Part model, mm, in its own coordinate system. Face numbers are marked on the shaded views. A direction names the side the tool comes from. Round coordinates to 2 decimals unless told otherwise and drop trailing zeros. Loops run counter-clockwise (first coordinate to the right, second up) from the corner with the lowest first, then second, coordinate; pieces in that order, holes last. Notation, with made-up numbers: (12, 82.25) -> (32, 82.25) arc R20 ccw to (32, 104.25) -> close; hole circle Ø3 at (-31.75, 84.25). An arc over 180 degrees is marked (long way). Use a Markdown table: item, result. Add a question column.
Item 1: Which spindle directions (+Z, -Z, +X, -X, +Y, -Y) get a long thin tool onto all of the face, cutting with end or side? Do the marked faces 1 and 2. Say none if no direction does.
Item 2: Cut at C-C, the plane y = 73. List the corners of the cut face in (x, z).
Item 3: Cut at B-B, the plane x = 12.5. List the corners of the cut face in (y, z).
Item 4: Flat gauge pins, fed straight in: pin 1 (6.5 mm diameter, centred on x = 0, z = 1.5, fed in from -Y); pin 2 (3 mm diameter, centred on y = 39.5, z = 6, fed in from -X); pin 3 (3.5 mm diameter, centred on x = 0, y = -6, fed in from +Z). Where does each tip first touch, or does it go through?
Item 5: Cut at D-D, the plane z = 5. List the corners of the cut face in (x, y), plus the area to 3 significant figures.
Item 6: Cut at A-A, the plane z = 0. List the corners of the cut face in (x, y).
Item 7: Probe line 1 (Z direction, x = -10, y = 64); line 2 (Y direction, x = 11.5, z = -2); line 3 (Z direction, x = -11, y = 67). List the from-to ranges inside material, lowest first. Write a range as [from, to].
```python
from build123d import *

# Parameters (mm, degrees)
ESQUISSE2_R             = 6
BOSS_EXTRU_1_DEPTH      = 1.5
ESQUISSE3_R             = 2.5
BOSS_EXTRU_2_DEPTH      = 10.5
TROU_TARAUD_M31_D       = 2.5
TROU_TARAUD_M31_DEPTH   = 4.5
TROU_TARAUD_M31_TIP     = 0.751075774
ESQUISSE7_W             = 4
ESQUISSE7_H             = 1.800245102
ENL_V_MAT_EXTRU_1_DEPTH = 9.5
ESQUISSE8_W             = 3
ESQUISSE8_H             = 0.5
BOSS_EXTRU_3_DEPTH      = 9.5


with BuildPart() as part:
    # Esquisse1 → R_volution1 (revolve)
    with BuildSketch(Plane.XY, mode=Mode.PRIVATE) as r_volution1_sk:
        Polygon((16, 0.5), (4, 0.5), (4, 0), (0, 0), (0, 67.3), (17.55, 67.3), (17.55, 43.5), (16, 43.5), align=None)
    revolve(r_volution1_sk.sketch.rotate(Axis((0, 0, 0), (0, 1, 0)), 90), axis=Axis((0, 0, 0), (0, 1, 0)))

    # Esquisse2 → Boss.-Extru.1 (add)
    with BuildSketch(Plane(origin=(0, 67.3, 0), x_dir=(1, 0, 0), z_dir=(0, 1, 0))):
        with Locations(Location((0, -8.73, 0), (0, 0, 270))):
            Circle(ESQUISSE2_R)
    extrude(amount=BOSS_EXTRU_1_DEPTH)

    # Esquisse3 → Boss.-Extru.2 (add)
    with BuildSketch(Plane(origin=(0, 68.8, 0), x_dir=(1, 0, 0), z_dir=(0, 1, 0))):
        with Locations(Location((0, -8.73, 0), (0, 0, 90))):
            Circle(ESQUISSE3_R)
    extrude(amount=BOSS_EXTRU_2_DEPTH)

    # Trou taraud_ M31
    with Locations(Plane(origin=(0, 67.3, 0), x_dir=(1, 0, 0), z_dir=(0, 1, 0))):
        with Locations((0, 13.37), (10.25, -8.73), (-10.25, -8.73)):
            Hole(TROU_TARAUD_M31_D / 2, depth=TROU_TARAUD_M31_DEPTH)
            with Locations((0, 0, -(TROU_TARAUD_M31_DEPTH + TROU_TARAUD_M31_TIP / 2))):  # 118° drill point
                Cone(0, TROU_TARAUD_M31_D / 2, TROU_TARAUD_M31_TIP, mode=Mode.SUBTRACT)

    # Esquisse7 → Enl_v. mat.-Extru.1 (cut)
    with BuildSketch(Plane(origin=(0, 79.3, 0), x_dir=(1, 0, 0), z_dir=(0, 1, 0))):
        with Locations((0, -11.130122551)):
            Rectangle(ESQUISSE7_W, ESQUISSE7_H)
    extrude(amount=-ENL_V_MAT_EXTRU_1_DEPTH, mode=Mode.SUBTRACT)

    # Esquisse8 → Boss.-Extru.3 (add)
    with BuildSketch(Plane.XZ.offset(-0.5)):
        with Locations((0, -11.25)):
            Rectangle(ESQUISSE8_W, ESQUISSE8_H)
        with Locations((0, 11.25)):
            Rectangle(ESQUISSE8_W, ESQUISSE8_H)
    extrude(amount=BOSS_EXTRU_3_DEPTH)


solid = part.part
```
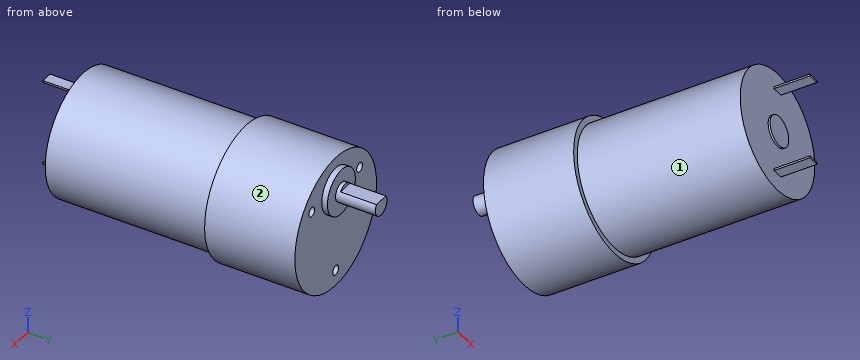
A:
| question | item | result |
|---|---|---|
| 1 | face 1 | -Y |
| 1 | face 2 | +Y, -Y |
| 2 | outline | (-2, 10.23) arc R2.5 ccw (long way) to (2, 10.23) -> close |
| 3 | outline | (0.5, -9.99) -> (43.5, -9.99) -> (43.5, -12.32) -> (67.3, -12.32) -> (67.3, 12.32) -> (43.5, 12.32) -> (43.5, 9.99) -> (0.5, 9.99) -> close |
| 4 | pin 1 | stops at y = 0 |
| 4 | pin 2 | stops at x = -15.35 |
| 4 | pin 3 | stops at z = 11.5 |
| 5 | outline | (-16.82, 43.5) -> (-15.2, 43.5) -> (-15.2, 0.5) -> (15.2, 0.5) -> (15.2, 43.5) -> (16.82, 43.5) -> (16.82, 67.3) -> (4.7, 67.3) -> (4.7, 68.8) -> (-4.7, 68.8) -> (-4.7, 67.3) -> (-16.82, 67.3) -> close |
| 5 | area | 2,120 mm^2 |
| 6 | outline | (-17.55, 43.5) -> (-16, 43.5) -> (-16, 0.5) -> (-4, 0.5) -> (-4, 0) -> (4, 0) -> (4, 0.5) -> (16, 0.5) -> (16, 43.5) -> (17.55, 43.5) -> (17.55, 67.3) -> (-17.55, 67.3) -> close |
| 7 | line 1 | z = [-14.42, 7.51], [9.95, 14.42] |
| 7 | line 2 | y = [0.5, 67.3] |
| 7 | line 3 | z = [-13.67, 7.73], [9.73, 13.67] |
